Geometry check sheet. Reference: the model listing, model coordinates, mm. A direction names the side the tool comes from. Round coordinates to 2 decimals unless told otherwise and drop trailing zeros. Loops run counter-clockwise (first coordinate to the right, second up) from the corner with the lowest first, then second, coordinate; pieces in that order, holes last. Notation, with made-up numbers: (63.5, 12.25) - (118.5, 12.25) arc R14 cw to (118.5, 37.25) - close; hole circle Ø6 at (3, 72.5). An arc over 180 degrees is marked (long way). Answer in a Markdown table with one row per item. Add a question column.
```python
from build123d import *

# Parameters (mm, degrees)
F1_DEPTH = 70
F2_R     = 1.95
F3_DEPTH = 25


with BuildPart() as f1:
    # F0 (on Front) → F1 (new body)
    with BuildSketch(Plane.XZ):
        Polygon((-5, 0.25), (-5, -2.75), (5, -2.75), (5, 0.25), (2.115, 0.25), (2, 0.25), (2, 2.75), (0, 2.75), (-2, 2.75), (-2, 0.25), align=None)
    extrude(amount=F1_DEPTH)

    # F2 (on face) → F3 (cut)
    with BuildSketch(Plane.XY.offset(2.75)):
        with Locations((0, -35)):
            Circle(F2_R)
    extrude(amount=-F3_DEPTH, mode=Mode.SUBTRACT)


solid = f1.part
```
Q1. Set-up check for faces 4 (the flat face through (-5, -35, -1)), 5 (the flat face through (4, -35, 0.25)), 6 (the flat face through (-3, -35, 0.25)): record each of +Z, -Z, +X, -X, +Y, -Y from which the full face is reachable in a straight line by a thin tool's end or side.
Q2. Release check for a two-part mould opening along Y. For faces 1 (the flat face through (0, 0, -1)), 2 (the cylindrical face through (1.048, -33.356, 0.038)), 3 (the flat face through (2.2, -34.5, -2.75)) record: +Y half, -Y half, draft (parallel to the pull), parting line (faces both ways), or undercut.
Q3. Cross-section at B-B, the plane y = -35. Enter the section's corners in (x, z), plus the area to 4 significant figures.
Q4. Scan lines: line 1 (Y direction, x = 0, z = -1.1); line 2 (Z direction, x = 2.25, y = -16); line 3 (Y direction, x = -1.5, z = -1.25). Record each from-to range of solid material in increasing order. Write a range as from..to.
Q5. Cross-section at A-A, the plane x = 0. Enter the section's corners in (y, z), plus the area to 3 significant figures.
Q6. Cross-section at D-D, the plane y = -24. Enter the section's corners in (x, z), plus the area to 3 significant figures.
Q7. Cross-section at C-C, the plane z = 1.05. Enter the section's corners in (x, y), plus the area to 3 significant figures.
Q8. Depth check by flat-ended pin: P1, Ø3, axis at y = -37.5, z = 1, coming from the -X side; P2, Ø1.5, axis at x = -3.5, y = -23.5, coming from the +Z side; P3, Ø2, axis at y = -61, z = 2, coming from the -X side. Enter the tip coordinate at first touch or a pass-through.
Check sheet entries:
| question | item | result |
|---|---|---|
| 1 | face 4 | +Z, -Z, -X, +Y, -Y |
| 1 | face 5 | +Z, +X, +Y, -Y |
| 1 | face 6 | +Z, -X, +Y, -Y |
| 2 | face 1 | +Y half |
| 2 | face 2 | undercut |
| 2 | face 3 | draft |
| 3 | outline | (-5, -2.75) - (-1.95, -2.75) - (-1.95, 2.75) - (-2, 2.75) - (-2, 0.25) - (-5, 0.25) - close; (1.95, -2.75) - (5, -2.75) - (5, 0.25) - (2, 0.25) - (2, 2.75) - (1.95, 2.75) - close |
| 3 | area | 18.55 mm² |
| 4 | line 1 | -70..-36.95, -33.05..0 |
| 4 | line 2 | -2.75..0.25 |
| 4 | line 3 | -70..-36.25, -33.75..0 |
| 5 | outline | (-70, -2.75) - (-36.95, -2.75) - (-36.95, 2.75) - (-70, 2.75) - close; (-33.05, -2.75) - (0, -2.75) - (0, 2.75) - (-33.05, 2.75) - close |
| 5 | area | 364 mm² |
| 6 | outline | (-5, -2.75) - (5, -2.75) - (5, 0.25) - (2, 0.25) - (2, 2.75) - (-2, 2.75) - (-2, 0.25) - (-5, 0.25) - close |
| 6 | area | 40.0 mm² |
| 7 | outline | (-2, -70) - (2, -70) - (2, 0) - (-2, 0) - close; hole circle Ø3.9 at (0, -35) |
| 7 | area | 268 mm² |
| 8 | P1 | x = -5 |
| 8 | P2 | z = 0.25 |
| 8 | P3 | x = -2 |
